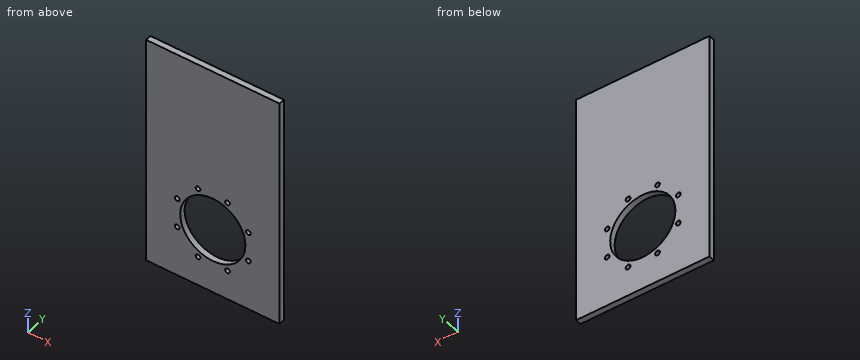
```python
from build123d import *

# Parameters (mm, degrees)
SKETCH1_W           = 225
SKETCH1_H           = 220
SKETCH1_R           = 55
BOSS_EXTRUDE1_DEPTH = 10
SKETCH2_R           = 4
CUT_EXTRUDE1_DEPTH  = 10
SKETCH3_W           = 225
SKETCH3_H           = 10
BOSS_EXTRUDE2_DEPTH = 169


with BuildPart() as part:
    # Sketch1 → Boss-Extrude1 (new body)
    with BuildSketch(Plane(origin=(0, 0, 0), x_dir=(1, 0, 0), z_dir=(0, 1, 0))):
        Rectangle(SKETCH1_W, SKETCH1_H)
        with Locations(Location((0, 0, 0), (0, 0, 270))):
            Circle(SKETCH1_R, mode=Mode.SUBTRACT)
    extrude(amount=BOSS_EXTRUDE1_DEPTH)

    # Sketch2 → Cut-Extrude1 (cut)
    with BuildSketch(Plane(origin=(0, 0, 0), x_dir=(1, 0, 0), z_dir=(0, 1, 0))):
        with Locations(Location((-24.874423104, -60.052169613, 0), (0, 0, 270))):
            Circle(SKETCH2_R)
        with Locations(Location((-60.052169613, -24.874423104, 0), (0, 0, 270))):
            Circle(SKETCH2_R)
        with Locations(Location((-60.052169613, 24.874423104, 0), (0, 0, 270))):
            Circle(SKETCH2_R)
        with Locations(Location((-24.874423104, 60.052169613, 0), (0, 0, 270))):
            Circle(SKETCH2_R)
        with Locations(Location((24.874423104, 60.052169613, 0), (0, 0, 270))):
            Circle(SKETCH2_R)
        with Locations(Location((60.052169613, 24.874423104, 0), (0, 0, 270))):
            Circle(SKETCH2_R)
        with Locations(Location((60.052169613, -24.874423104, 0), (0, 0, 270))):
            Circle(SKETCH2_R)
        with Locations(Location((24.874423104, -60.052169613, 0), (0, 0, 270))):
            Circle(SKETCH2_R)
    extrude(amount=CUT_EXTRUDE1_DEPTH, mode=Mode.SUBTRACT)

    # Sketch3 → Boss-Extrude2 (add)
    with BuildSketch(Plane.XY.offset(110)):
        with Locations((0, 5)):
            Rectangle(SKETCH3_W, SKETCH3_H)
    extrude(amount=BOSS_EXTRUDE2_DEPTH)


solid = part.part
```
CAD build for the part. Positions are in the model's coordinates, mm. Round coordinates to 2 decimals unless told otherwise and drop trailing zeros. Loops run counter-clockwise (first coordinate to the right, second up) from the corner with the lowest first, then second, coordinate; pieces in that order, holes last. Notation, with made-up numbers: (7.25, 57.25) - (38.25, 57.25) arc R26 ccw to (38.25, 83.25) - close; hole circle Ø1 at (0, 45). An arc over 180 degrees is marked (long way). Return JSON: item names as keys, results as strings. Group by question number.
Q1. Band-saw the part on C-C on y = 8.25. Give the number of separate pieces and of enclosed holes in the cut face, plus the area to 3 significant figures.
Q2. Band-saw the part on B-B on z = 0. Give the cut face in (x, y).
Q3. Band-saw the part on A-A on x = 0. Give the cut face in (y, z).
Q4. Drill centre lines: line 1 along X through (y, z) = (9.5, 27); line 2 along X through (y, z) = (4.5, 58); line 3 along Z through (x, y) = (45.5, 3.25). Where is each one in solid material? Low to high. Write a range as [from, to].
Solutions:
{
 "1": {"separate pieces": "1", "enclosed holes": "9", "area": "77,600 mm^2"},
 "2": {"outline": "(-112.5, 0) - (-55, 0) - (-55, 10) - (-112.5, 10) - close; (55, 0) - (112.5, 0) - (112.5, 10) - (55, 10) - close"},
 "3": {"outline": "(0, -110) - (10, -110) - (10, -55) - (0, -55) - close; (0, 55) - (10, 55) - (10, 279) - (0, 279) - close"},
 "4": {"line 1": "x = [-112.5, -63.44], [-56.66, -47.92], [47.92, 56.66], [63.44, 112.5]", "line 2": "x = [-112.5, -28.31], [-21.44, 21.44], [28.31, 112.5]", "line 3": "z = [-110, -30.9], [30.9, 279]"}
}
